from build123d import *

# Parameters (mm, degrees)
SKETCH_W        = 105
SKETCH_H        = 193
PAD_DEPTH       = 5
SKETCH001_R     = 1.5
POCKET_DEPTH    = 5.001
SKETCH003_W     = 53
SKETCH003_H     = 141
POCKET002_DEPTH = 5.001
FILLET_R        = 4


with BuildPart() as part:
    # Sketch → Pad (new body)
    with BuildSketch(Plane.XY):
        Rectangle(SKETCH_W, SKETCH_H)
    extrude(amount=PAD_DEPTH)

    # Sketch001 (on Face6 of Pad) → Pocket (cut, through all)
    with BuildSketch(Plane.XY.offset(5)):
        with Locations((-44.5, 86)):
            Circle(SKETCH001_R)
        with Locations((44.5, 86)):
            Circle(SKETCH001_R)
        with Locations((-44.5, -86)):
            Circle(SKETCH001_R)
        with Locations((44.5, -86)):
            Circle(SKETCH001_R)
    extrude(amount=-POCKET_DEPTH, mode=Mode.SUBTRACT)

    # Sketch003 → Pocket002 (cut, through all)
    with BuildSketch(Plane.XY):
        Rectangle(SKETCH003_W, SKETCH003_H)
    extrude(amount=POCKET002_DEPTH, mode=Mode.SUBTRACT)

    # Fillet
    fillet_edges = [part.edges().sort_by_distance(p)[0] for p in [
        (-52.5, 96.5, 2.5),
        (-52.5, -96.5, 2.5),
        (52.5, -96.5, 2.5),
        (52.5, 96.5, 2.5),
        (26.5, 70.5, 2.5),
        (26.5, -70.5, 2.5),
        (-26.5, -70.5, 2.5),
        (-26.5, 70.5, 2.5),
    ]]
    fillet(fillet_edges, radius=FILLET_R)


solid = part.part
Check sheet for the modelled part. Datum: model origin and axes. Units: mm. A direction names the side the tool comes from. Give positions to 0.01 mm unless a question says otherwise; leave off trailing zeros. Loops run counter-clockwise (first coordinate to the right, second up) from the corner with the lowest first, then second, coordinate; pieces in that order, holes last. Notation, with made-up numbers: M 77,26 L 103,26 A19 ccw 103,55 Z; hole C 1.5,-13.5 d7. An arc over 180 degrees is marked long. Answer as a JSON object with one key per item and string values. Group by question number.
Q1. Access from +Z, -Z, +X, -X, +Y, -Y to the whole of each face (thin tool, end or side, straight path). Record for faces 5 (the cylindrical face through (-25.297, 69.359, 2.535)), 6 (the flat face through (-52.5, -1, 2)).
Q2. Cross-section at B-B on x = 1. Record the cut outline in (y, z), then the cut area to 3 significant figures.
Q3. Material ranges on line 1 along X through (y, z) = (-86, 2.3); line 2 along X through (y, z) = (-65, 1.3); line 3 along Y through (x, z) = (-44.5, 3), recorded low to high. Write a range as [from, to].
Q4. Cross-section at C-C on z = 2.7. Record the cut outline in (x, y).
Q5. Cross-section at A-A on y = 16.5. Record the cut outline in (x, z), then the cut area to 3 significant figures.
Q6. Go/stop test with a flat-tipped pin: P1, Ø3.5, axis at x = -44.5, y = 86, coming from the -Z side. Record where the tip stops, or that it passes through.
Q7. Release check for a two-part mould opening along X. For faces 1 (the flat face through (52.5, -1, 2)), 2 (the flat face through (0, 70.5, 2)), 3 (the flat face through (-1, 96.5, 2)), 4 (the cylindrical face through (-51.359, -95.297, 2.535)) record: released by +X, released by -X, zero draft, split by the parting line, or undercut.
Evaluation:
{
 "1": {"face 5": "+Z, -Z", "face 6": "+Z, -Z, -X, +Y, -Y"},
 "2": {"outline": "M -96.5,0 L -70.5,0 L -70.5,5 L -96.5,5 Z; M 70.5,0 L 96.5,0 L 96.5,5 L 70.5,5 Z", "area": "260 mm2"},
 "3": {"line 1": "x = [-52.5, -46], [-43, 43], [46, 52.5]", "line 2": "x = [-52.5, -26.5], [26.5, 52.5]", "line 3": "y = [-96.5, -87.5], [-84.5, 84.5], [87.5, 96.5]"},
 "4": {"outline": "M -52.5,-92.5 A4 ccw -48.5,-96.5 L 48.5,-96.5 A4 ccw 52.5,-92.5 L 52.5,92.5 A4 ccw 48.5,96.5 L -48.5,96.5 A4 ccw -52.5,92.5 Z; hole C -44.5,-86 d3; hole C -44.5,86 d3; hole M -26.5,-66.5 A4 ccw -22.5,-70.5 L 22.5,-70.5 A4 ccw 26.5,-66.5 L 26.5,66.5 A4 ccw 22.5,70.5 L -22.5,70.5 A4 ccw -26.5,66.5 Z; hole C 44.5,-86 d3; hole C 44.5,86 d3"},
 "5": {"outline": "M -52.5,0 L -26.5,0 L -26.5,5 L -52.5,5 Z; M 26.5,0 L 52.5,0 L 52.5,5 L 26.5,5 Z", "area": "260 mm2"},
 "6": {"P1": "stops at z = 0"},
 "7": {"face 1": "released by +X", "face 2": "undercut", "face 3": "zero draft", "face 4": "released by -X"}
}
